Build history of the part. All positions in model axes, mm. Round coordinates to 2 decimals unless told otherwise and drop trailing zeros. Loops run counter-clockwise (first coordinate to the right, second up) from the corner with the lowest first, then second, coordinate; pieces in that order, holes last. Notation, with made-up numbers: (71, 22.25) -> (124, 22.25) arc R13 cw to (124, 30.25) -> close; hole circle Ø7 at (46.25, -19.75). An arc over 180 degrees is marked (long way). Put each result on its own line as item: value. Start each with the question number.
```python
from build123d import *

# Parameters (mm, degrees)
SKETCH2_R = 1.7653


with BuildPart() as part:
    # Sweep1: sweep along a path in Sketch1
    with BuildLine(Plane(origin=(0, 0, 0), x_dir=(1, 0, 0), z_dir=(0, 1, 0))) as sweep1_path:
        Line((-142.799128817, 75.082728817), (142.799128817, 75.082728817))
        ThreePointArc((142.799128817, 75.082728817), (157.778196027, 68.878196027), (163.982728817, 53.899128817))
        Line((163.982728817, 53.899128817), (163.982728817, -53.899128817))
        ThreePointArc((163.982728817, -53.899128817), (157.778196027, -68.878196027), (142.799128817, -75.082728817))
        Line((142.799128817, -75.082728817), (-142.799128817, -75.082728817))
        ThreePointArc((-142.799128817, -75.082728817), (-157.778196027, -68.878196027), (-163.982728817, -53.899128817))
        Line((-163.982728817, -53.899128817), (-163.982728817, 53.899128817))
        ThreePointArc((-163.982728817, 53.899128817), (-157.778196027, 68.878196027), (-142.799128817, 75.082728817))
    # Sketch2 → Sweep1 (sweep)
    with BuildSketch(Plane(origin=(0, 0, 0), x_dir=(0, 0, -1), z_dir=(1, 0, 0))):
        with Locations((-76.848028817, 0)):
            Circle(SKETCH2_R)
    sweep(path=sweep1_path.line)


solid = part.part
```
Item 1: Cut at B-B on x = 96.5. Write the cut outline in (y, z).
Item 2: Cut at A-A on y = 0. Write the cut outline in (x, z).
Item 3: Cut at C-C on z = 4.5. Write the cut outline in (x, y), then the cut area to 3 significant figures.
Item 4: Wall check: line 1 (Z direction, x = -100, y = -0.5); line 2 (X direction, y = 0.5, z = 3.5); line 3 (Z direction, x = 5.5, y = 0.1). Give the ranges that are in metal, low to high. Write a range as from..to.
Item 5: Drop flat-ended pins along their axis: pin 1 (1 mm diameter, centred on x = 117, y = 1, fed in from +Z); pin 2 (2 mm diameter, centred on y = -1, z = 51.5, fed in from -X); pin 3 (1.5 mm diameter, centred on y = 1.5, z = 42, fed in from +X). Give the stop position or say it passes through.
Ans:
1. outline: circle Ø3.53 at (0, -76.85); circle Ø3.53 at (0, 76.85)
2. outline: (-167.51, -53.9) arc R24.71 ccw to (-142.8, -78.61) -> (142.8, -78.61) arc R24.71 ccw to (167.51, -53.9) -> (167.51, 53.9) arc R24.71 ccw to (142.8, 78.61) -> (-142.8, 78.61) arc R24.71 ccw to (-167.51, 53.9) -> close; hole (-163.98, -53.9) arc R21.18 ccw to (-142.8, -75.08) -> (142.8, -75.08) arc R21.18 ccw to (163.98, -53.9) -> (163.98, 53.9) arc R21.18 ccw to (142.8, 75.08) -> (-142.8, 75.08) arc R21.18 ccw to (-163.98, 53.9) -> close
3. outline: circle Ø3.53 at (-165.75, 0); circle Ø3.53 at (165.75, 0)
3. area: 19.6 mm2
4. line 1: z = -78.54..-75.16, 75.16..78.54
4. line 2: x = -167.44..-164.06, 164.06..167.44
4. line 3: z = -78.61..-75.09, 75.09..78.61
5. pin 1: stops at z = 78.54
5. pin 2: stops at x = -167.51
5. pin 3: stops at x = 167.35
